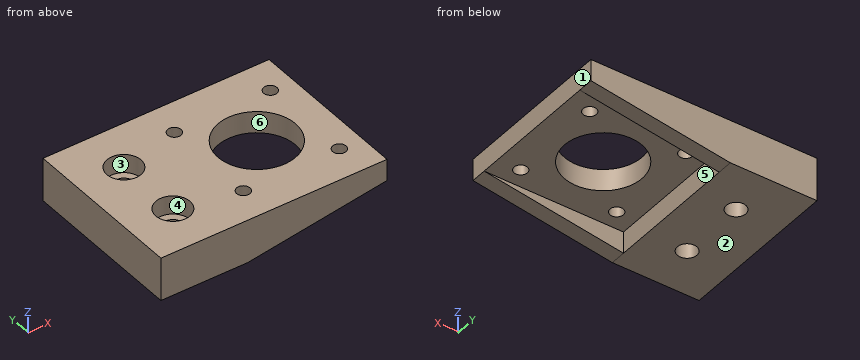
```python
from build123d import *

# Parameters (mm, degrees)
F0_W     = 73
F0_H     = 43
F0_R     = 3.15
F0_R_2   = 2.15
F0_R_3   = 12.5
F1_DEPTH = 20
F2_W     = 73
F2_H     = 6
F2_W_2   = 45
F2_H_2   = 7
F3_DEPTH = 43.001
F4_W     = 73
F4_H     = 5
F5_DEPTH = 14
F7_DEPTH = 53.001
F8_R     = 5.5
F9_DEPTH = 6


with BuildPart() as f1:
    # F0 (on Top) → F1 (new body)
    with BuildSketch(Plane.XY):
        Rectangle(F0_W, F0_H)
        with Locations((-21.5, -11)):
            Circle(F0_R, mode=Mode.SUBTRACT)
        with Locations((-2, -15.5)):
            Circle(F0_R_2, mode=Mode.SUBTRACT)
        with Locations((29, -15.5)):
            Circle(F0_R_2, mode=Mode.SUBTRACT)
        with Locations((-21.5, 11)):
            Circle(F0_R, mode=Mode.SUBTRACT)
        with Locations((-2, 15.5)):
            Circle(F0_R_2, mode=Mode.SUBTRACT)
        with Locations((13.5, 0)):
            Circle(F0_R_3, mode=Mode.SUBTRACT)
        with Locations((29, 15.5)):
            Circle(F0_R_2, mode=Mode.SUBTRACT)
    extrude(amount=F1_DEPTH)

    # F2 (on face) → F3 (cut, through all)
    with BuildSketch(Plane.XZ.offset(21.5)):
        with Locations((0, 17)):
            Rectangle(F2_W, F2_H)
        with Locations((14, 3.5)):
            Rectangle(F2_W_2, F2_H_2)
    extrude(amount=-F3_DEPTH, mode=Mode.SUBTRACT)

    # F4 (on face) → F5 (join, through all)
    with BuildSketch(Plane.XY.offset(14)):
        with Locations((0, -24)):
            Rectangle(F4_W, F4_H)
        with Locations((0, 24)):
            Rectangle(F4_W, F4_H)
    extrude(amount=-F5_DEPTH)

    # F6 (on face) → F7 (cut, through all)
    with BuildSketch(Plane.XZ.offset(26.5)):
        Polygon((36.5, 7), (-8.5, 0), (36.5, 0), align=None)
    extrude(amount=-F7_DEPTH, mode=Mode.SUBTRACT)

    # F8 (on face) → F9 (cut)
    with BuildSketch(Plane.XY.offset(14)):
        with Locations((-21.5, 11)):
            Circle(F8_R)
        with Locations((-21.5, -11)):
            Circle(F8_R)
    extrude(amount=-F9_DEPTH, mode=Mode.SUBTRACT)


solid = f1.part
```
Check sheet for the modelled part. Datum: model origin and axes. Units: mm. Face numbers are marked on the shaded views. A direction names the side the tool comes from. Give positions to 0.01 mm unless a question says otherwise; leave off trailing zeros. Order: outer loops, then holes, each group sorted by start corner. A loop starts at its lowest first (then second) coordinate and runs counter-clockwise, first axis right, second up. Notation, with made-up numbers: M 34.25,-22 L 47.25,-22 A14 cw 47.25,-13 Z; hole C 31.5,10 d8. An arc over 180 degrees is marked long. Answer in a Markdown table with one row per item. Add a question column.
Q1. Sectioned sample at B-B, the plane z = 9.5. Record the boundary of the cut face in (x, y).
Q2. Access from +Z, -Z, +X, -X, +Y, -Y to the whole of each face (thin tool, end or side, straight path). Record for the marked faces 4, 5 and 6.
Q3. Gauge pin test, flat ends, axial feed: pin 1 Ø6 at (x, y) = (19, -18) entering from -Z; pin 2 Ø12.5 at (x, y) = (-21.5, 11) entering from +Z; pin 3 Ø3.5 at (x, z) = (20.5, 2.5) entering from +Y; pin 4 Ø8 at (x, y) = (-21.5, -11) entering from +Z. Record the tip position at first contact, or that the pin passes through.
Q4. Sectioned sample at D-D, the plane y = 11. Record the boundary of the cut face in (x, z).
Q5. Thickness scan on L1, parallel to Y at x = -2, z = 12.25; L2, parallel to Y at x = -21.5, z = 6.5; L3, parallel to Y at x = 27, z = 6. Record the ranges inside material, lowest first.
Q6. Release check for a two-part mould opening along X. For the marked faces 1, 2 and 3 record: released by +X, released by -X, zero draft, split by the parting line, or undercut.
Q7. Sectioned sample at C-C, the plane x = 13.5. Record the boundary of the cut face in (y, z), and give its area (3 significant figures).
Q8. Sectioned sample at A-A, the plane y = 0. Record the boundary of the cut face in (x, z), and give its area (3 significant figures).
Verdict:
| question | item | result |
|---|---|---|
| 1 | outline | M -36.5,-26.5 L 36.5,-26.5 L 36.5,26.5 L -36.5,26.5 Z; hole C -21.5,-11 d11; hole C -21.5,11 d11; hole C -2,-15.5 d4.3; hole C -2,15.5 d4.3; hole C 13.5,0 d25; hole C 29,-15.5 d4.3; hole C 29,15.5 d4.3 |
| 2 | face 4 | +Z |
| 2 | face 5 | -Z, +X |
| 2 | face 6 | +Z, -Z |
| 3 | pin 1 | z = 7 |
| 3 | pin 2 | z = 14 |
| 3 | pin 3 | through |
| 3 | pin 4 | z = 8 |
| 4 | outline | M -36.5,0 L -24.65,0 L -24.65,8 L -27,8 L -27,14 L -36.5,14 Z; M -18.35,0 L -8.5,0 L -8.5,7 L 7.56,7 L 7.56,14 L -16,14 L -16,8 L -18.35,8 Z; M 19.44,7 L 36.5,7 L 36.5,14 L 19.44,14 Z |
| 5 | L1 | -26.5 to -17.65, -13.35 to 13.35, 17.65 to 26.5 |
| 5 | L2 | -26.5 to -14.15, -7.85 to 7.85, 14.15 to 26.5 |
| 5 | L3 | -26.5 to -21.5, 21.5 to 26.5 |
| 6 | face 1 | released by +X |
| 6 | face 2 | zero draft |
| 6 | face 3 | undercut |
| 7 | outline | M -26.5,3.42 L -21.5,3.42 L -21.5,7 L -12.5,7 L -12.5,14 L -26.5,14 Z; M 12.5,7 L 21.5,7 L 21.5,3.42 L 26.5,3.42 L 26.5,14 L 12.5,14 Z |
| 7 | area | 232 mm² |
| 8 | outline | M -36.5,0 L -8.5,0 L -8.5,7 L 1,7 L 1,14 L -36.5,14 Z; M 26,7 L 36.5,7 L 36.5,14 L 26,14 Z |
| 8 | area | 532 mm² |
